Verification items for the finished model (mm, model axes). A direction names the side the tool comes from. Give positions to 0.01 mm unless a question says otherwise; leave off trailing zeros. Loops run counter-clockwise (first coordinate to the right, second up) from the corner with the lowest first, then second, coordinate; pieces in that order, holes last. Notation, with made-up numbers: (76.5, 7) - (107.5, 7) arc R23 ccw to (107.5, 15) - close; hole circle Ø10 at (53.25, 86.5). An arc over 180 degrees is marked (long way). One line per question, with ' | ' between items. Start each with the question number.
1. Section check B-B, the plane z = 2.9. Enter the section's corners in (x, y).
2. Section check D-D, the plane y = 1.75. Enter the section's corners in (x, z), then the cut area to 3 significant figures.
3. Depth check by flat-ended pin: pin 1 Ø1 at (x, z) = (0, 2.9) entering from +Y; pin 2 Ø3 at (x, y) = (-5, 2) entering from -Z; pin 3 Ø1.5 at (y, z) = (-2.5, 4) entering from -X. Enter the tip coordinate at first touch or a pass-through.
4. Section check C-C, the plane z = 1.35. Enter the section's corners in (x, y), then the cut area to 3 significant figures.
5. Tool access check on faces 1 (the face through (-2.7, 1.59, 2.86)), 2 (the face through (-0.141, 4.402, 3.535)). Record the directions out of +Z, -Z, +X, -X, +Y, -Y that give a thin tool (end or side, any length) a straight path to the whole face; none if there is none.
6. Mould release check, pull along Y, two halves, no side actions. Record for faces 3 (the face through (4.857, 2.857, 2.859)), 4 (the face through (2.7, -1.59, 2.86)), 5 (the face through (4.9, -2.78, 2.86)): +Y half, -Y half, draft (parallel to the pull), parting line (faces both ways), or undercut.
7. Section check A-A, the plane x = 0. Enter the section's corners in (y, z), then the cut area to 3 significant figures.
8. Thickness scan on line 1 along Y through (x, z) = (0, 2.1); line 2 along Z through (x, y) = (0, 4.6); line 3 along X through (y, z) = (-4.25, 2.9). Record the ranges inside material, lowest first. Write a range as from..to.
Autodesk Inventor part; units mm, degrees
ref_plane "YZ Plane" through (0, 0, 0) normal (1, 0, 0) x (0, 1, 0)
ref_plane "XZ Plane" through (0, 0, 0) normal (0, 1, 0) x (-1, 0, 0)
ref_plane "XY Plane" through (0, 0, 0) normal (0, 0, 1) x (1, 0, 0)
sketch "Sketch5" plane through (0, 0, 0) normal (0, 0, 1) x (1, 0, 0)
  line L0 (0, 0) -> (3.1, 0) construction
  circle A0 centre (0, 0) radius 3.1 construction
  line L1 (0, 0) -> (1.55, 2.6847) construction
  line L2 (0, 0) -> (-1.55, 2.6847) construction
  line L3 (0, 0) -> (-3.1, 0) construction
  line L4 (0, 0) -> (-1.55, -2.6847) construction
  line L5 (0, 0) -> (1.55, -2.6847) construction
  line L6 (-1.55, 2.6847) -> (1.55, 2.6847) construction
  line L7 (1.55, 2.6847) -> (3.1, 0) construction
  line L8 (3.1, 0) -> (1.55, -2.6847) construction
  line L9 (-1.55, 2.6847) -> (-3.1, 0) construction
  line L10 (-3.1, 0) -> (-1.55, -2.6847) construction
  line L11 (-1.55, -2.6847) -> (1.55, -2.6847) construction
  line L12 (3.6196, 0) -> (1.8098, 3.1347)
  line L13 (1.8098, 3.1347) -> (-1.8098, 3.1347)
  line L14 (-1.8098, 3.1347) -> (-3.6196, 0)
  line L15 (-3.6196, 0) -> (-1.8098, -3.1347)
  line L16 (-1.8098, -3.1347) -> (1.8098, -3.1347)
  line L17 (1.8098, -3.1347) -> (3.6196, 0)
  line L18 (3.2532, 5.6347) -> (6.5064, 0)
  line L19 (6.5064, 0) -> (3.2532, -5.6347)
  line L20 (3.2532, -5.6347) -> (-3.2532, -5.6347)
  line L21 (-3.2532, -5.6347) -> (-6.5064, 0)
  line L22 (-6.5064, 0) -> (-3.2532, 5.6347)
  line L23 (-3.2532, 5.6347) -> (3.2532, 5.6347)
  dimension "d9" = 3.1
  dimension "d12" = 360
  dimension "d14" = 0.45
  dimension "d15" = 2.5
extrude "Extrusion4" add sketch "Sketch5" along normal blind 5.8
sketch "Sketch6" plane through (-3.2532, 5.6347, 0) normal (0, 1, 0) x (1, 0, 0)
  line L0 (0, -5.8) -> (6.5064, -5.8)
  line L1 (3.2532, -5.8) -> (3.2532, 0) construction
  line L2 (0, 0) -> (0, -5.8)
  line L3 (0, -2.9) -> (6.5064, -2.9) construction
  line L4 (6.5064, 0) -> (6.5064, -5.8)
  circle A0 centre (3.2532, -2.9) radius 0.65
  dimension "d18" = 1.3
extrude "Extrusion5" cut sketch "Sketch6" against normal blind 15
properties part number "Hombro_Ejes"
Results list:
1) outline: (-6.51, 0) - (-3.25, -5.63) - (-0.65, -5.63) - (-0.65, -3.13) - (-1.81, -3.13) - (-3.62, 0) - (-1.81, 3.13) - (-0.65, 3.13) - (-0.65, 5.63) - (-3.25, 5.63) - close; (0.65, -5.63) - (3.25, -5.63) - (6.51, 0) - (3.25, 5.63) - (0.65, 5.63) - (0.65, 3.13) - (1.81, 3.13) - (3.62, 0) - (1.81, -3.13) - (0.65, -3.13) - close
2) outline: (-5.5, 0) - (-2.61, 0) - (-2.61, 5.8) - (-5.5, 5.8) - close; (2.61, 0) - (5.5, 0) - (5.5, 5.8) - (2.61, 5.8) - close | area: 33.5 mm²
3) pin 1: through | pin 2: z = 0 | pin 3: x = -5.5
4) outline: (-6.51, 0) - (-3.25, -5.63) - (3.25, -5.63) - (6.51, 0) - (3.25, 5.63) - (-3.25, 5.63) - close; hole (-3.62, 0) - (-1.81, -3.13) - (1.81, -3.13) - (3.62, 0) - (1.81, 3.13) - (-1.81, 3.13) - close | area: 75.9 mm²
5) face 1: +Z, -Z | face 2: +Y, -Y
6) face 3: +Y half | face 4: undercut | face 5: -Y half
7) outline: (-5.63, 0) - (-3.13, 0) - (-3.13, 2.25) - (-5.63, 2.25) - close; (-5.63, 3.55) - (-3.13, 3.55) - (-3.13, 5.8) - (-5.63, 5.8) - close; (3.13, 0) - (5.63, 0) - (5.63, 2.25) - (3.13, 2.25) - close; (3.13, 3.55) - (5.63, 3.55) - (5.63, 5.8) - (3.13, 5.8) - close | area: 22.5 mm²
8) line 1: -5.63..-3.13, 3.13..5.63 | line 2: 0..2.25, 3.55..5.8 | line 3: -4.05..-0.65, 0.65..4.05
